```python
from build123d import *

# Parameters (mm, degrees)
SKETCH1_W           = 89
SKETCH1_H           = 30
BOSS_EXTRUDE1_DEPTH = 94
BOSS_EXTRUDE2_DEPTH = 94
CUT_EXTRUDE2_START  = 5
SKETCH4_W           = 178
SKETCH4_H           = 59.703545047
CUT_EXTRUDE2_DEPTH  = 150
SKETCH5_R           = 2
SKETCH5_R_2         = 1.5
CUT_EXTRUDE3_DEPTH  = 10
FILLET1_R           = 100
FILLET2_R           = 50
FILLET3_R           = 40
BOSS_EXTRUDE3_DEPTH = 5
SKETCH8_R           = 2.25
CUT_EXTRUDE5_DEPTH  = 5
FILLET4_R           = 40
SKETCH10_R          = 1.25
SKETCH10_R_2        = 5
CUT_EXTRUDE6_DEPTH  = 5
CHAMFER1_SIZE       = 1
SKETCH11_R          = 4
CUT_EXTRUDE7_DEPTH  = 2


with BuildPart() as part:
    # Sketch1 → Boss-Extrude1 (new, symmetric)
    with BuildSketch(Plane.XY):
        with Locations((44.5, 15)):
            Rectangle(SKETCH1_W, SKETCH1_H)
    extrude(amount=BOSS_EXTRUDE1_DEPTH, both=True)

    # Sketch2 → Boss-Extrude2 (add, symmetric)
    with BuildSketch(Plane.XY):
        with BuildLine():
            Line((75.771243445, 0), (102.228756555, 0))
            ThreePointArc((102.228756555, 0), (89, 35), (75.771243445, 0))
        make_face()
    extrude(amount=BOSS_EXTRUDE2_DEPTH, both=True)

    # Sketch4 → Cut-Extrude2 (cut)
    with BuildSketch(Plane(origin=(0, 0, 0), x_dir=(0, 0, -1), z_dir=(1, 0, 0)).offset(CUT_EXTRUDE2_START)):
        with Locations((0, 25.910589708)):
            Rectangle(SKETCH4_W, SKETCH4_H)
    extrude(amount=CUT_EXTRUDE2_DEPTH, mode=Mode.SUBTRACT)

    # Sketch5 → Cut-Extrude3 (cut)
    with BuildSketch(Plane(origin=(0, 0, -94), x_dir=(-1, 0, 0), z_dir=(0, 0, -1))):
        with Locations((-89, 15)):
            Circle(SKETCH5_R)
        with Locations((-95, 15)):
            Circle(SKETCH5_R_2)
        with Locations((-89, 21)):
            Circle(SKETCH5_R_2)
        with Locations((-83, 15)):
            Circle(SKETCH5_R_2)
        with Locations((-89, 9)):
            Circle(SKETCH5_R_2)
    extrude(amount=-CUT_EXTRUDE3_DEPTH, mode=Mode.SUBTRACT)

    # Fillet1
    fillet1_edges = [part.edges().sort_by_distance(p)[0] for p in [
        (75.771243445, 30, -91.5),
        (75.771243445, 30, 91.5),
    ]]
    fillet(fillet1_edges, radius=FILLET1_R)

    # Fillet2
    fillet2_edges = [part.edges().sort_by_distance(p)[0] for p in [
        (5, 15, -89),
        (5, 15, 89),
    ]]
    fillet(fillet2_edges, radius=FILLET2_R)

    # Fillet3
    fillet3_edges = [part.edges().sort_by_distance(p)[0] for p in [
        (0, 15, 94),
        (0, 15, -94),
    ]]
    fillet(fillet3_edges, radius=FILLET3_R)

    # Sketch7 → Boss-Extrude3 (add)
    with BuildSketch(Plane.ZY):
        with BuildLine():
            Line((-16.770509831, 0), (16.770509831, 0))
            ThreePointArc((16.770509831, 0), (0, 37.5), (-16.770509831, 0))
        make_face()
    extrude(amount=-BOSS_EXTRUDE3_DEPTH)

    # Sketch8 → Cut-Extrude5 (cut)
    with BuildSketch(Plane(origin=(0, 0, 89), x_dir=(-1, 0, 0), z_dir=(0, 0, -1))):
        with Locations(Location((-89, 15, 0), (0, 0, 90))):
            Circle(SKETCH8_R)
    extrude(amount=-CUT_EXTRUDE5_DEPTH, mode=Mode.SUBTRACT)

    # Fillet4
    fillet4_edges = [part.edges().sort_by_distance(p)[0] for p in [
        (2.5, 30, 16.770509831),
        (2.5, 30, -16.770509831),
    ]]
    fillet(fillet4_edges, radius=FILLET4_R)

    # Sketch10 → Cut-Extrude6 (cut)
    with BuildSketch(Plane.ZY):
        with Locations((-13.856406461, 7)):
            Circle(SKETCH10_R)
        with Locations((0, 31)):
            Circle(SKETCH10_R)
        with Locations((13.856406461, 7)):
            Circle(SKETCH10_R)
        with Locations((0, 15)):
            Circle(SKETCH10_R_2)
    extrude(amount=-CUT_EXTRUDE6_DEPTH, mode=Mode.SUBTRACT)

    # Chamfer1
    chamfer1_edges = [part.edges().sort_by_distance(p)[0] for p in [
        (96.5, 15, -89),
        (90.5, 21, -89),
        (84.5, 15, -89),
        (90.5, 9, -89),
    ]]
    chamfer(chamfer1_edges, length=CHAMFER1_SIZE)

    # Sketch11 → Cut-Extrude7 (cut)
    with BuildSketch(Plane(origin=(0, 0, 89), x_dir=(-1, 0, 0), z_dir=(0, 0, -1))):
        with Locations((-89, 15)):
            Circle(SKETCH11_R)
    extrude(amount=-CUT_EXTRUDE7_DEPTH, mode=Mode.SUBTRACT)


solid = part.part
```
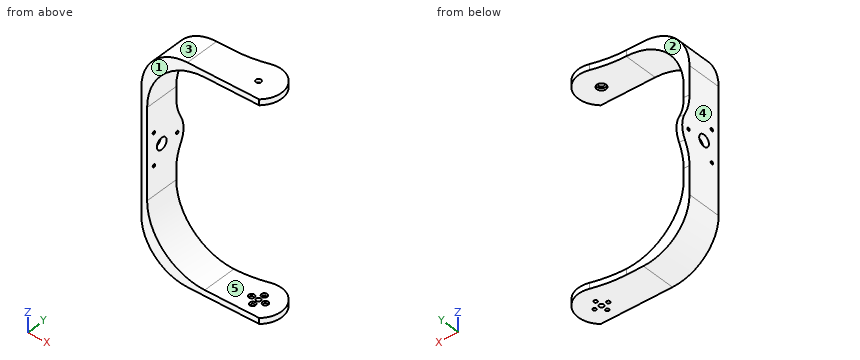
Geometry: final body of the model. Coordinates: model frame, mm. Face numbers are marked on the shaded views. A direction names the side the tool comes from. Round coordinates to 2 decimals unless told otherwise and drop trailing zeros. Write each loop counter-clockwise with the first axis right and the second up, starting at its lowest first coordinate (ties: lowest second). Pieces come first, ordered by that corner, then holes. Notation, with made-up numbers: (87, 79.25) -> (107, 79.25) arc R20 ccw to (107, 87.25) -> close; hole circle Ø7 at (-28, -8.75). An arc over 180 degrees is marked (long way). Use CSV: the item, a comma, the result in double quotes. Start each with the question number.
Q1. First-contact query: pin 1 Ø1.5 at (y, z) = (7, 13.86) entering from +X; pin 2 Ø12 at (y, z) = (19.5, 13.5) entering from +X; pin 3 Ø8 at (y, z) = (30, 65) entering from -X; pin 4 Ø1.8 at (x, y) = (95, 15) entering from -Z. Flat tips, straight axial feed; report the tip coordinate or a pass-through.
Q2. Section C-C (z = -47). Return loops of the section in (x, y), plus the area to 3 significant figures.
Q3. Line query: L1, parallel to Y at x = 2.7, z = 0; L2, parallel to Z at x = 80, y = 3.5; L3, parallel to Y at x = 89, z = 89.5. Output: solid intervals per line, ascending.
Q4. Section D-D (z = 23.5). Return loops of the section in (x, y).
Q5. Pull-direction query (Y, two-part tool) for the marked faces 1, 2 and 3; classes: pulls with the +Y half, pulls with the -Y half, needs draft (parallel to the pull), parting line crosses it, or undercut.
Q6. Section A-A (x = 69). Return loops of the section in (y, z).
Q7. Section B-B (y = 26). Return loops of the section in (x, z), plus the area to 3 significant figures.
Q8. Reachability of the marked faces 4 and 5 from +Z, -Z, +X, -X, +Y, -Y: full face, straight path, thin tool, end or side. Return the list, or none.
Result sheet:
1,pin 1,"through"
1,pin 2,"x = 5"
1,pin 3,"x = 0.62"
1,pin 4,"z = 89"
2,outline,"(0, 0) -> (5.64, 0) -> (5.64, 30) -> (0, 30) -> close"
2,area,"169 mm²"
3,L1,"0 to 10, 20 to 29.75, 32.25 to 37.5"
3,L2,"-94 to -89, 89 to 94"
3,L3,"0 to 11, 19 to 35"
4,outline,"(0, 0) -> (5, 0) -> (5, 30.48) -> (0, 30.48) -> close"
5,face 1,"pulls with the -Y half"
5,face 2,"pulls with the +Y half"
5,face 3,"needs draft"
6,outline,"(0, -94) -> (31.02, -94) -> (31.02, -89) -> (0, -89) -> close; (0, 89) -> (31.02, 89) -> (31.02, 94) -> (0, 94) -> close"
7,outline,"(0, -54) arc R40 ccw to (40, -94) -> (105.7, -94) -> (105.7, -89) -> (55, -89) arc R50 cw to (5, -39) -> (5, 39) arc R50 cw to (55, 89) -> (105.7, 89) -> (105.7, 94) -> (40, 94) arc R40 ccw to (0, 54) -> close"
7,area,"2,330 mm²"
8,face 4,"+Z, -Z, -X, +Y, -Y"
8,face 5,"+X, +Y, -Y"
